Read the model definition and answer for the solid it produces. Units are mm, in the model's axes. A direction names the side the tool comes from. Coordinates: 2 decimals unless noted, no trailing zeros. Loops run counter-clockwise (first coordinate to the right, second up) from the corner with the lowest first, then second, coordinate; pieces in that order, holes last. Notation, with made-up numbers: M -7,-16 L 4,-16 A27 cw 4,4 Z; hole C 79.25,3.5 d3. An arc over 180 degrees is marked long. Use one line per item in the form item = value. Start each with the question number.
1. The part is cut by section D-D (z = 0). Give the vertices of the cut face in (x, y), plus the area to 3 significant figures.
2. The part is cut by section C-C (y = 20). Give the vertices of the cut face in (x, z).
3. Find the intervals of material crossed by probe 1 along Z at (x, y) = (-11, 0); probe 2 along X at (y, z) = (18.5, 3); probe 3 along Y at (x, z) = (4.5, -1), in increasing order. Write a range as [from, to].
4. The part is cut by section A-A (y = 0). Give the vertices of the cut face in (x, z), plus the area to 3 significant figures.
5. A tool of negligible diameter and unlimited length cuts with its end or side. For faces 5 (the flat face through (7, 17.7, -0.1)), 6 (the flat face through (-3, 19.8, -2.3)), 7 (the cylindrical face through (9.73, 3.06, -0.07)), from which of +Z, -Z, +X, -X, +Y, -Y can it reach the whole face along a straight path? Write none if from no direction.
6. For a pull along Y with two mould halves and no side action, classify faces 1 (the flat face through (2, 25, 0)), 2 (the cylindrical face through (12.536, -1.774, 0.923)), 3 (the flat face through (3, 10, -5)), 4 (the cylindrical face through (2, 22, 0)) as released by +Y, released by -Y, zero draft, split by the parting line, or undercut.
7. Flat-ended cylindrical pins translate along their axes: pin 1 (2.5 mm diameter, centred on y = 0, z = 0, fed in from +X); pin 2 (6 mm diameter, centred on x = -7.5, z = -2.5, fed in from -Y); pin 3 (1 mm diameter, centred on y = 7, z = -0.5, fed in from +X); pin 4 (3 mm diameter, centred on y = 12.5, z = 1.5, fed in from -X). Find the tip coordinate at first contact, or state that the pin passes through.
8. The part is cut by section B-B (x = 0). Give the vertices of the cut face in (y, z).
from build123d import *

# Parameters (mm, degrees)
CYLINDER003_R     = 2
CYLINDER003_DEPTH = 10
CYLINDER004_R     = 2
CYLINDER004_DEPTH = 30
CYLINDER001_R     = 10.2
CYLINDER001_DEPTH = 10
BOX_W             = 10
BOX_H             = 15
BOX_DEPTH         = 10
CYLINDER_R        = 15
CYLINDER_DEPTH    = 10


with BuildPart() as cylinder003:
    # Cylinder003 → Cylinder003 (new body)
    with BuildSketch(Plane(origin=(7, 20, 0), x_dir=(0, 0, 1), z_dir=(-1, 0, 0))):
        Circle(CYLINDER003_R)
    extrude(amount=CYLINDER003_DEPTH)


with BuildPart() as cylinder004:
    # Cylinder004 → Cylinder004 (new body)
    with BuildSketch(Plane.ZY.offset(-15)):
        Circle(CYLINDER004_R)
    extrude(amount=CYLINDER004_DEPTH)


with BuildPart() as negative_fusion:
    # Cylinder001 → Cylinder001 (new body)
    with BuildSketch(Plane.XY.offset(-5)):
        Circle(CYLINDER001_R)
    extrude(amount=CYLINDER001_DEPTH)

    # Fusion: union Cylinder003, Cylinder004
    add(cylinder003.part)
    add(cylinder004.part)


with BuildPart() as cube:
    # Box → Box (new body)
    with BuildSketch(Plane(origin=(-3, 10, -5), x_dir=(1, 0, 0), z_dir=(0, 0, 1))):
        with Locations((5, 7.5)):
            Rectangle(BOX_W, BOX_H)
    extrude(amount=BOX_DEPTH)


with BuildPart() as cut:
    # Cylinder → Cylinder (new body)
    with BuildSketch(Plane.XY.offset(-5)):
        Circle(CYLINDER_R)
    extrude(amount=CYLINDER_DEPTH)

    # Fusion001: union Cube
    add(cube.part)

    # Cut: cut Negative Fusion
    add(negative_fusion.part, mode=Mode.SUBTRACT)


solid = cut.part
Computed values:
q1.outline = M -14.87,-2 A15 ccw 14.87,-2 L 10,-2 A10.2 cw -10,-2 Z; M -14.87,2 L -10,2 A10.2 cw 10,2 L 14.87,2 A15 ccw 7,13.27 L 7,18 L -3,18 L -3,14.7 A15 ccw Z; M -3,22 L 7,22 L 7,25 L -3,25 Z
q1.area = 406 mm²
q2.outline = M -3,-5 L 7,-5 L 7,-2 L -3,-2 Z; M -3,2 L 7,2 L 7,5 L -3,5 Z
q3.probe_1 = [-5, -2], [2, 5]
q3.probe_2 = [-3, 7]
q3.probe_3 = [-14.31, -9.15], [9.15, 18.27], [21.73, 25]
q4.outline = M -15,-5 L -10.2,-5 L -10.2,-2 L -15,-2 Z; M -15,2 L -10.2,2 L -10.2,5 L -15,5 Z; M 10.2,-5 L 15,-5 L 15,-2 L 10.2,-2 Z; M 10.2,2 L 15,2 L 15,5 L 10.2,5 Z
q4.area = 57.6 mm²
q5.face_5 = +Z, -Z, +X, +Y
q5.face_6 = +Z, -Z, -X, +Y
q5.face_7 = +Z, -Z
q6.face_1 = released by +Y
q6.face_2 = undercut
q6.face_3 = zero draft
q6.face_4 = undercut
q7.pin_1 = through
q7.pin_2 = -14.31
q7.pin_3 = 13.52
q7.pin_4 = -10.2
q8.outline = M -15,-5 L -10.2,-5 L -10.2,5 L -15,5 Z; M 10.2,-5 L 25,-5 L 25,5 L 10.2,5 Z; hole C 20,0 d4
